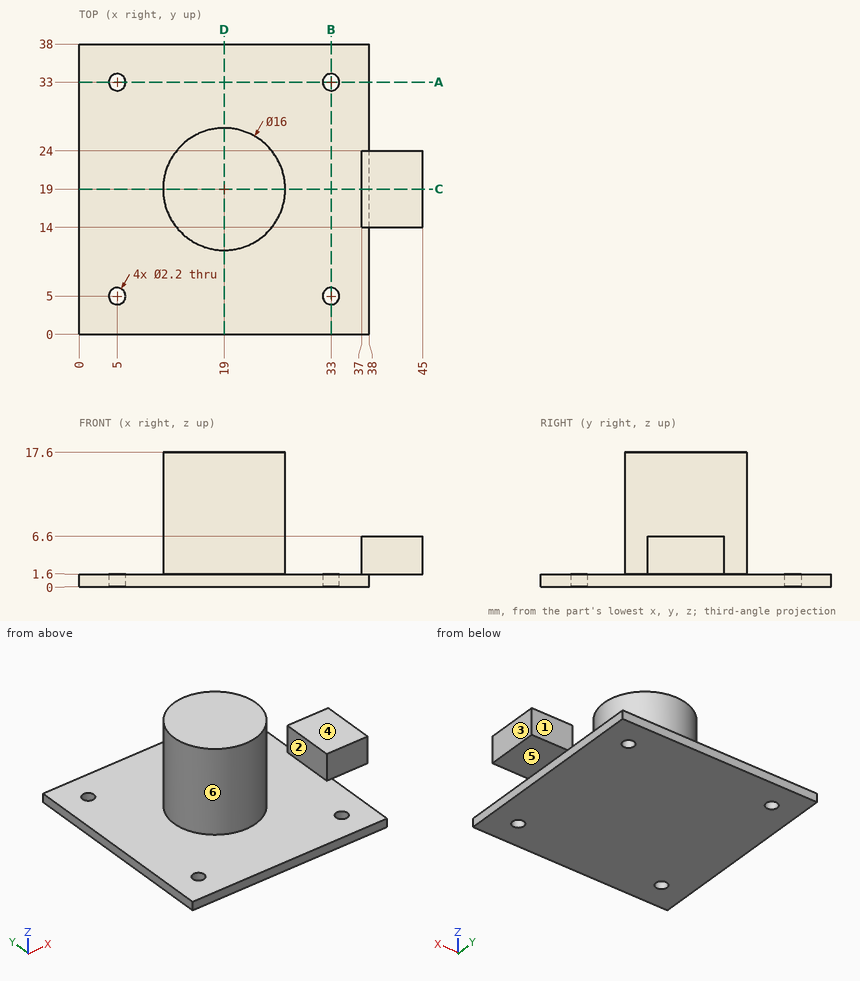
The drawing under review shows one solid part. Ordinate dimensions are in mm from its lowest x, y, z. A direction names the side the tool comes from. Round coordinates to 2 decimals unless told otherwise and drop trailing zeros. Loops run counter-clockwise (first coordinate to the right, second up) from the corner with the lowest first, then second, coordinate; pieces in that order, holes last. Notation, with made-up numbers: M 79.25,62.5 L 97.25,62.5 A12 cw 97.25,85.5 Z; hole C 89,52 d11. An arc over 180 degrees is marked long. Answer as CSV lines item,"result". Start each with the question number.
Item 1: Consider section D-D (x = 19). Write out the cut boundary in (y, z).
Item 2: Mouldability with a two-part tool opening along X and no side actions: class the marked faces 1, 2 and 3 as released by +X, released by -X, zero draft, split by the parting line, or undercut.
Item 3: Insertion check: P1, Ø1, axis at x = 5.5, z = 3.5, coming from the -Y side; P2, Ø6, axis at y = 11.5, z = 7.5, coming from the -X side; P3, Ø1.5, axis at x = 40.5, z = 4.5, coming from the +Y side; P4, Ø0.8, axis at y = 20.5, z = 1, coming from the +X side. Each pin has a flat end and moves straight along its axis. Give the tip position at first contact, or say it passes through.
Item 4: Consider section C-C (y = 19). Write out the cut boundary in (x, z).
Item 5: Consider section A-A (y = 33). Write out the cut boundary in (x, z), then the cut area to 3 significant figures.
Item 6: For the marked faces 4, 5 and 6, list the 3-axis set-ups (+Z, -Z, +X, -X, +Y, -Y) from which the entire face can be reached by the end or side of a thin tool; tool diameter is ignored.
Item 7: Wall thickness on line 1 (X direction, y = 33, z = 0.55); line 2 (Z direction, x = 13, y = 28.5): over which ranges is each line inside the solid? List them lowest first. Write a range as [from, to].
Answer:
1,outline,"M 0,0 L 38,0 L 38,1.6 L 27,1.6 L 27,17.6 L 11,17.6 L 11,1.6 L 0,1.6 Z"
2,face 1,"zero draft"
2,face 2,"undercut"
2,face 3,"released by +X"
3,P1,"passes through"
3,P2,"stops at x = 12.39"
3,P3,"stops at y = 24"
3,P4,"stops at x = 38"
4,outline,"M 0,0 L 38,0 L 38,1.6 L 45,1.6 L 45,6.6 L 37,6.6 L 37,1.6 L 27,1.6 L 27,17.6 L 11,17.6 L 11,1.6 L 0,1.6 Z"
5,outline,"M 0,0 L 3.9,0 L 3.9,1.6 L 0,1.6 Z; M 6.1,0 L 31.9,0 L 31.9,1.6 L 6.1,1.6 Z; M 34.1,0 L 38,0 L 38,1.6 L 34.1,1.6 Z"
5,area,"53.8 mm^2"
6,face 4,"+Z, +X, +Y, -Y"
6,face 5,"-Z, +X, +Y, -Y"
6,face 6,"+Z"
7,line 1,"x = [0, 3.9], [6.1, 31.9], [34.1, 38]"
7,line 2,"z = [0, 1.6]"
